Input: dimensioned drawing with shaded views. Units: mm. Origin: part minimum x, y, z. Give positions to 0.01 mm unless a question says otherwise; leave off trailing zeros. Write each loop counter-clockwise with the first axis right and the second up, starting at its lowest first coordinate (ties: lowest second). Pieces come first, ordered by that corner, then holes. Notation, with made-up numbers: (39, 81.25) - (89, 81.25) arc R7 cw to (89, 92.25) - close; hole circle Ø3 at (-26.75, 66.25). An arc over 180 degrees is marked (long way). Answer as a JSON object with one key per item and string values. Group by question number.
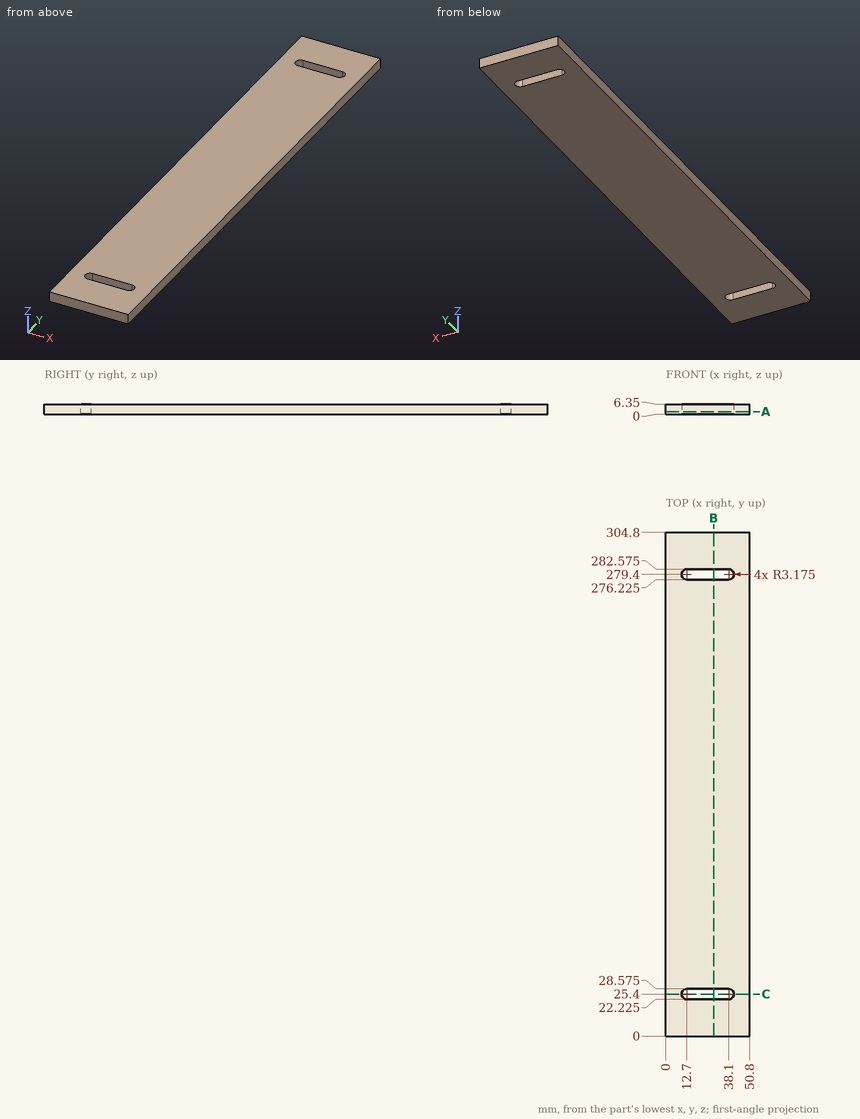
Q1. Section C-C on y = 25.4. Return the cut outline in (x, z) (3 decimals).
Q2. Section B-B on x = 29. Return the cut outline in (y, z) (3 decimals).
Q3. Ray query, probe 1 along Y at (x, z) = (25.5, 2.5) (3 decimals); probe 2 along Y at (x, z) = (10, 5.5). Return the intervals inside material, ascending. Write a range as [from, to].
Q4. Section A-A on z = 1.75. Return the cut outline in (x, y) (3 decimals), then the cut area to 3 significant figures.
Taken from the geometry:
{
 "1": {"outline": "(0, 0) - (9.525, 0) - (9.525, 6.35) - (0, 6.35) - close; (41.275, 0) - (50.8, 0) - (50.8, 6.35) - (41.275, 6.35) - close"},
 "2": {"outline": "(0, 0) - (22.225, 0) - (22.225, 6.35) - (0, 6.35) - close; (28.575, 0) - (276.225, 0) - (276.225, 6.35) - (28.575, 6.35) - close; (282.575, 0) - (304.8, 0) - (304.8, 6.35) - (282.575, 6.35) - close"},
 "3": {"probe 1": "y = [0, 22.225], [28.575, 276.225], [282.575, 304.8]", "probe 2": "y = [0, 23.73], [27.07, 277.73], [281.07, 304.8]"},
 "4": {"outline": "(0, 0) - (50.8, 0) - (50.8, 304.8) - (0, 304.8) - close; hole (12.7, 22.225) - (38.1, 22.225) arc R3.175 ccw to (38.1, 28.575) - (12.7, 28.575) arc R3.175 ccw to start; hole (12.7, 276.225) - (38.1, 276.225) arc R3.175 ccw to (38.1, 282.575) - (12.7, 282.575) arc R3.175 ccw to start", "area": "15,100 mm²"}
}
